Design review of the part built by this model. Coordinates are the model's own, in mm. Give positions to 0.01 mm unless a question says otherwise; leave off trailing zeros. Write each loop counter-clockwise with the first axis right and the second up, starting at its lowest first coordinate (ties: lowest second). Pieces come first, ordered by that corner, then holes.
```python
from build123d import *

# Parameters (mm, degrees)
F0_R     = 3.175
F1_DEPTH = 3.048


with BuildPart() as f1:
    # F0 (on Front) → F1 (new body)
    with BuildSketch(Plane.XZ):
        with BuildLine():
            ThreePointArc((0.124512, 47.944903), (0.093353, 48.939042), (0, 49.929278))
            ThreePointArc((0, 49.929278), (-15.750488, 63.819903), (-31.500977, 49.929278))
            ThreePointArc((-31.500977, 49.929278), (-31.617878, 48.436388), (-31.593595, 46.939124))
            ThreePointArc((-31.593595, 46.939124), (-15.750488, 32.069903), (0.092619, 46.939124))
            ThreePointArc((0.092619, 46.939124), (0.116536, 47.441761), (0.124512, 47.944903))
        make_face()
        with Locations((-15.750488, 47.944903)):
            Circle(F0_R, mode=Mode.SUBTRACT)
        with BuildLine():
            ThreePointArc((-6.300195, 99.935528), (-6.244183, 99.341386), (-6.225488, 98.744903))
            ThreePointArc((-6.225488, 98.744903), (-16.346972, 89.238598), (-25.200781, 99.935528))
            Line((-25.200781, 99.935528), (-31.500977, 49.929278))
            ThreePointArc((-31.500977, 49.929278), (-15.750488, 63.819903), (0, 49.929278))
            Line((0, 49.929278), (-6.300195, 99.935528))
        make_face()
        with Locations((-18.925488, 84.470103)):
            Circle(F0_R, mode=Mode.SUBTRACT)
        with BuildLine():
            ThreePointArc((-25.200781, 99.935528), (-16.346972, 89.238598), (-6.225488, 98.744903))
            ThreePointArc((-6.225488, 98.744903), (-6.244183, 99.341386), (-6.300195, 99.935528))
            ThreePointArc((-6.300195, 99.935528), (-15.750488, 108.269903), (-25.200781, 99.935528))
        make_face()
        with Locations((-15.750488, 98.744903)):
            Circle(F0_R, mode=Mode.SUBTRACT)
        with BuildLine():
            ThreePointArc((-3.898602, -15.555097), (-16.126122, -3.709165), (-27.578564, -16.305987))
            ThreePointArc((-27.578564, -16.305987), (-23.472446, -24.546124), (-14.70678, -27.360938))
            ThreePointArc((-14.70678, -27.360938), (-7.266757, -23.831178), (-3.922413, -16.305987))
            ThreePointArc((-3.922413, -16.305987), (-3.904557, -15.930731), (-3.898602, -15.555097))
        make_face()
        with Locations((-15.750488, -15.555097)):
            Circle(F0_R, mode=Mode.SUBTRACT)
        with BuildLine():
            ThreePointArc((0.092619, 46.939124), (-15.750488, 32.069903), (-31.593595, 46.939124))
            Line((-31.593595, 46.939124), (-27.578564, -16.305987))
            ThreePointArc((-27.578564, -16.305987), (-16.126122, -3.709165), (-3.898602, -15.555097))
            ThreePointArc((-3.898602, -15.555097), (-3.904557, -15.930731), (-3.922413, -16.305987))
            ThreePointArc((-3.922413, -16.305987), (-7.266757, -23.831178), (-14.70678, -27.360938))
            Line((-14.70678, -27.360938), (29.398509, -23.461759))
            ThreePointArc((29.398509, -23.461759), (20.762012, -15.555097), (29.398509, -7.648435))
            Line((29.398509, -7.648435), (4.535575, -5.450399))
            ThreePointArc((4.535575, -5.450399), (-0.795456, -2.710945), (-2.698537, 2.972608))
            Line((-2.698537, 2.972608), (0.092619, 46.939124))
        make_face()
        with BuildLine():
            ThreePointArc((29.398509, -7.648435), (20.762012, -15.555097), (29.398509, -23.461759))
            ThreePointArc((29.398509, -23.461759), (34.554091, -20.91493), (36.637012, -15.555097))
            ThreePointArc((36.637012, -15.555097), (34.554091, -10.195264), (29.398509, -7.648435))
        make_face()
        with Locations((28.699512, -15.555097)):
            Circle(F0_R, mode=Mode.SUBTRACT)
    extrude(amount=F1_DEPTH)


solid = f1.part
```
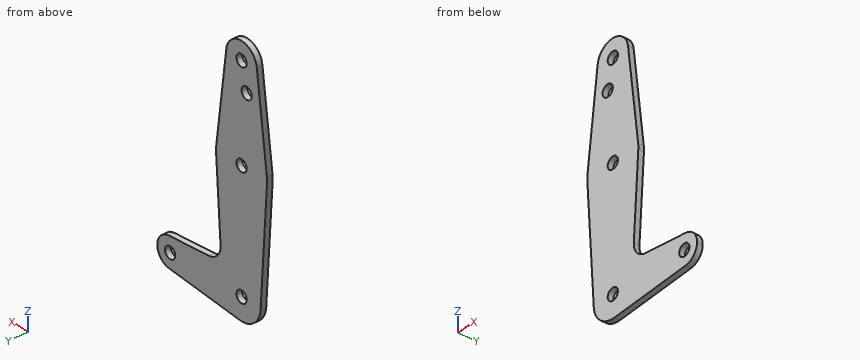
(1) Consider section A-A, the plane y = -2.2. Give the number of separate pieces and of enclosed holes in the cut face, then the cut area to 3 significant figures.
Resolved:
separate pieces: 1
enclosed holes: 5
area: 4,020 mm2
(2) To check wall thickness, follow L1, parallel to Z at x = -17.5, y = -2.6; L2, parallel to Z at x = 27.5, y = -2.35; L3, parallel to Z at x = 31.5, y = -0.2. State the ranges of each line that lie inside material, in increasing order.
Resolved:
L1: z = -27.28 to -18.2, -12.91 to 45.3, 50.59 to 81.63, 87.31 to 96.1, 101.39 to 108.11
L2: z = -23.63 to -18.49, -12.62 to -7.48
L3: z = -22.98 to -17.05, -14.06 to -8.13
(3) Consider section B-B, the plane z = 7. Give the boundary of the cut face in (x, y), then the cut area to 3 significant figures.
Resolved:
outline: (-29.06, -3.05) - (-2.44, -3.05) - (-2.44, 0) - (-29.06, 0) - close
area: 81.1 mm2
(4) Clearance check with flat-ended pins moving along their axes: P1, Ø5.5, axis at x = 28.7, z = -15.56, coming from the +Y side; P2, Ø1, axis at x = -21, y = -2, coming from the -Z side. State where each tip first meets the part, or that it passes through.
Resolved:
P1: passes through
P2: stops at z = -26.41
(5) Consider section C-C, the plane z = 32.5. Give the boundary of the cut face in (x, y).
Resolved:
outline: (-30.68, -3.05) - (-0.82, -3.05) - (-0.82, 0) - (-30.68, 0) - close
